from build123d import *

# Parameters (mm, degrees)
F0_W     = 41
F0_H     = 108
F1_DEPTH = 11


with BuildPart() as f1:
    # F0 (on Top) → F1 (new body)
    with BuildSketch(Plane.XY):
        with BuildLine():
            ThreePointArc((5.706968, -5.714822), (7.712615, -8.087528), (8.791989, -11.000826))
            ThreePointArc((8.791989, -11.000826), (11.232354, -10.554221), (12.600096, -12.624032))
            ThreePointArc((12.600096, -12.624032), (11.232354, -14.693844), (8.791989, -14.247239))
            ThreePointArc((8.791989, -14.247239), (7.713498, -17.159023), (5.709659, -19.530996))
            ThreePointArc((5.709659, -19.530996), (8.425965, -20.996255), (10.784891, -22.986424))
            ThreePointArc((10.784891, -22.986424), (13.862215, -18.206159), (14.939576, -12.624032))
            ThreePointArc((14.939576, -12.624032), (13.862843, -7.043472), (10.787222, -2.264082))
            ThreePointArc((10.787222, -2.264082), (8.425588, -4.252233), (5.706968, -5.714822))
        make_face()
        with BuildLine():
            ThreePointArc((-8.919726, -11.038862), (-7.830592, -8.082615), (-5.789315, -5.682866))
            ThreePointArc((-5.789315, -5.682866), (-8.499762, -4.205185), (-10.850307, -2.203935))
            ThreePointArc((-10.850307, -2.203935), (-15.060422, -12.616237), (-10.861132, -23.032909))
            ThreePointArc((-10.861132, -23.032909), (-8.510775, -21.032627), (-5.800788, -19.555715))
            ThreePointArc((-5.800788, -19.555715), (-7.814796, -17.19237), (-8.905782, -14.285245))
            ThreePointArc((-8.905782, -14.285245), (-12.720827, -12.678409), (-8.919726, -11.038862))
        make_face()
        with BuildLine():
            ThreePointArc((5.603682, 1.265457), (8.381963, -0.225399), (10.787222, -2.264082))
            ThreePointArc((10.787222, -2.264082), (13.905039, 2.536774), (14.997339, 8.156016))
            ThreePointArc((14.997339, 8.156016), (13.878906, 13.839509), (10.690392, 18.675455))
            ThreePointArc((10.690392, 18.675455), (8.324534, 16.666348), (5.595827, 15.187174))
            ThreePointArc((5.595827, 15.187174), (7.57988, 12.907076), (8.697198, 10.09871))
            ThreePointArc((8.697198, 10.09871), (11.379114, 10.5015), (12.850096, 8.223097))
            ThreePointArc((12.850096, 8.223097), (11.379114, 5.944693), (8.697198, 6.347483))
            ThreePointArc((8.697198, 6.347483), (7.582521, 3.543455), (5.603682, 1.265457))
        make_face()
        with BuildLine():
            ThreePointArc((-10.842957, 18.523657), (-15.00266, 8.161334), (-10.850307, -2.203935))
            ThreePointArc((-10.850307, -2.203935), (-8.49497, -0.220064), (-5.784132, 1.241002))
            ThreePointArc((-5.784132, 1.241002), (-7.772737, 3.510479), (-8.899446, 6.309695))
            ThreePointArc((-8.899446, 6.309695), (-13.060362, 8.167454), (-8.915558, 10.060887))
            ThreePointArc((-8.915558, 10.060887), (-7.810312, 12.874025), (-5.83607, 15.162624))
            ThreePointArc((-5.83607, 15.162624), (-8.510157, 16.588935), (-10.842957, 18.523657))
        make_face()
        with Locations((0, -1)):
            Rectangle(F0_W, F0_H)
        with BuildLine():
            ThreePointArc((14.997339, 8.156016), (13.905039, 2.536774), (10.787222, -2.264082))
            ThreePointArc((10.787222, -2.264082), (13.862843, -7.043472), (14.939576, -12.624032))
            ThreePointArc((14.939576, -12.624032), (13.862215, -18.206159), (10.784891, -22.986424))
            ThreePointArc((10.784891, -22.986424), (13.894801, -27.783287), (14.984183, -33.3953))
            ThreePointArc((14.984183, -33.3953), (-5.597944, -47.317938), (-10.861132, -23.032909))
            ThreePointArc((-10.861132, -23.032909), (-15.060422, -12.616237), (-10.850307, -2.203935))
            ThreePointArc((-10.850307, -2.203935), (-15.00266, 8.161334), (-10.842957, 18.523657))
            ThreePointArc((-10.842957, 18.523657), (-5.833397, 42.924664), (14.850096, 29.043097))
            ThreePointArc((14.850096, 29.043097), (13.771383, 23.457599), (10.690392, 18.675455))
            ThreePointArc((10.690392, 18.675455), (13.878906, 13.839509), (14.997339, 8.156016))
        make_face(mode=Mode.SUBTRACT)
    extrude(amount=F1_DEPTH)


solid = f1.part
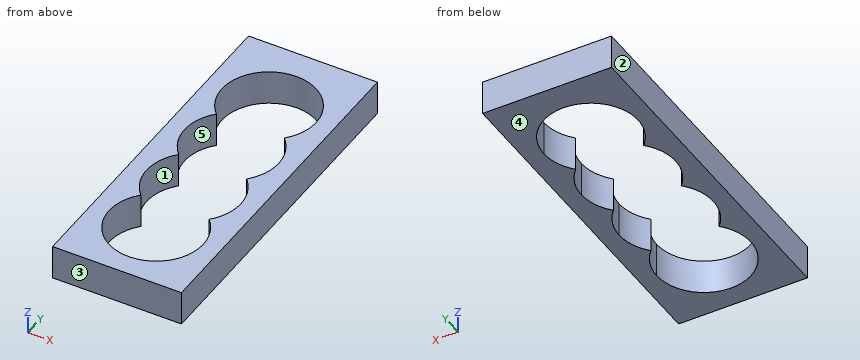
The listing builds one solid part. Answer for the finished solid, in the listing's coordinates (mm). Face numbers are marked on the shaded views. A direction names the side the tool comes from. Coordinates: 2 decimals unless noted, no trailing zeros. Write each loop counter-clockwise with the first axis right and the second up, starting at its lowest first coordinate (ties: lowest second). Pieces come first, ordered by that corner, then holes. Notation, with made-up numbers: (2, 59.5) -> (16, 59.5) arc R16 cw to (16, 77.5) -> close; hole circle Ø5 at (-39, -30.5). An arc over 180 degrees is marked (long way). One line per question, with ' | ' between items.
1. Section A-A (y = 39) is taken. Determine the outline of the cut face in (x, z), and give its area (3 significant figures).
Verdict:
outline: (-20.5, 0) -> (-11.37, 0) -> (-11.37, 11) -> (-20.5, 11) -> close; (11.07, 0) -> (20.5, 0) -> (20.5, 11) -> (11.07, 11) -> close | area: 204 mm^2
2. For a pull along Y with two mould halves and no side action, classify the marked faces 3, 4 and 5 as released by +Y, released by -Y, zero draft, split by the parting line, or undercut.
Verdict:
face 3: released by -Y | face 4: zero draft | face 5: undercut
3. Which of the six approach directions +Z, -Z, +X, -X, +Y, -Y give full straight-line access (tool end or side, diameter ignored) to the marked faces 1 and 2?
Verdict:
face 1: +Z, -Z | face 2: +Z, -Z, -X, +Y, -Y
4. Section B-B (x = 7.5) is taken. Determine the outline of the cut face in (y, z), and give its area (3 significant figures).
Verdict:
outline: (-55, 0) -> (-46.38, 0) -> (-46.38, 11) -> (-55, 11) -> close; (41.95, 0) -> (53, 0) -> (53, 11) -> (41.95, 11) -> close | area: 216 mm^2
5. Section C-C (z = 3) is taken. Determine the outline of the cut face in (x, y), and give its area (3 significant figures).
Verdict:
outline: (-20.5, -55) -> (20.5, -55) -> (20.5, 53) -> (-20.5, 53) -> close; hole (-10.86, -23.03) arc R15 ccw (long way) to (14.98, -33.4) arc R15 ccw to (10.78, -22.99) arc R15 ccw to (14.94, -12.62) arc R15 ccw to (10.79, -2.26) arc R15 ccw to (15, 8.16) arc R15 ccw to (10.69, 18.68) arc R15 ccw to (14.85, 29.04) arc R15 ccw (long way) to (-10.84, 18.52) arc R15 ccw to (-10.85, -2.2) arc R15 ccw to start | area: 2,010 mm^2
6. Straight lines are drawn through the part: line 1 (Y direction, x = 0.5, z = 6.25); line 2 (Y direction, x = 13, z = 5.75); line 3 (Y direction, x = -5, z = 1). For each, find the intervals that lie inside material, in ascending order.
Verdict:
line 1: y = -55 to -48.39, 44.03 to 53 | line 2: y = -55 to -40.85, -25.94 to -20, -5.25 to 0.68, 15.63 to 21.83, 36.26 to 53 | line 3: y = -55 to -47.54, 43.24 to 53
